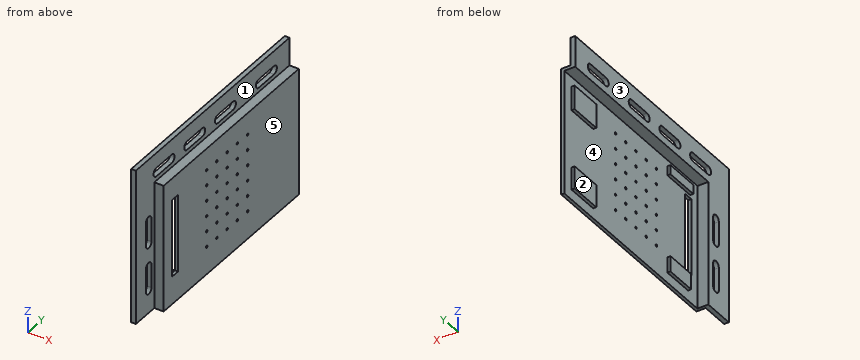
from build123d import *

# Parameters (mm, degrees)
EXTRUDE_1_DEPTH             = 3
EXTRUDE_2_DEPTH             = 6
EXTRUDE_3_DEPTH             = 3
SKETCH_5_W                  = 2
SKETCH_5_H                  = 80
EXTRUDE_4_DEPTH             = 130
SKETCH_6_W                  = 50
SKETCH_6_H                  = 6
CUT_EXTRUDE_1_DEPTH         = 130
SKETCH_7_W                  = 14.471008782
SKETCH_7_H                  = 21.149935912
SKETCH_7_W_2                = 15.39863755
SKETCH_7_W_3                = 10.018390695
SKETCH_7_H_2                = 20.222307144
SKETCH_7_W_4                = 5.936824115
SKETCH_7_H_3                = 22.263090434
EXTRUDE_5_DEPTH             = 2
SKETCH_8_R                  = 0.75
CUT_EXTRUDE_2_DEPTH         = 2
PATTERN_LINEAR_1_COUNT      = 5
PATTERN_LINEAR_1_PITCH      = 10
PATTERN_LINEAR_1_COUNT_DIR2 = 6
PATTERN_LINEAR_1_PITCH_DIR2 = 10


with BuildPart() as part:
    # Sketch 1 → Extrude 1 (new body)
    with BuildSketch(Plane(origin=(0, 0, 0), x_dir=(0, 0, -1), z_dir=(1, 0, 0))):
        Polygon((0, 0), (0, 150), (18, 150), (18, 18), (100, 18), (100, 0), align=None)
        with BuildLine():
            ThreePointArc((85, 9.75), (87.75, 12.5), (85, 15.25))
            Line((85, 15.25), (70, 15.25))
            ThreePointArc((70, 15.25), (67.25, 12.5), (70, 9.75))
            Line((70, 9.75), (85, 9.75))
        make_face(mode=Mode.SUBTRACT)
        with BuildLine():
            ThreePointArc((55, 9.75), (57.75, 12.5), (55, 15.25))
            Line((55, 15.25), (40, 15.25))
            ThreePointArc((40, 15.25), (37.25, 12.5), (40, 9.75))
            Line((40, 9.75), (55, 9.75))
        make_face(mode=Mode.SUBTRACT)
        with BuildLine():
            ThreePointArc((15.25, 135), (12.5, 137.75), (9.75, 135))
            Line((9.75, 135), (9.75, 120))
            ThreePointArc((9.75, 120), (12.5, 117.25), (15.25, 120))
            Line((15.25, 120), (15.25, 135))
        make_face(mode=Mode.SUBTRACT)
        with BuildLine():
            ThreePointArc((15.25, 95), (12.5, 97.75), (9.75, 95))
            Line((9.75, 95), (9.75, 80))
            ThreePointArc((9.75, 80), (12.5, 77.25), (15.25, 80))
            Line((15.25, 80), (15.25, 95))
        make_face(mode=Mode.SUBTRACT)
        with BuildLine():
            ThreePointArc((15.25, 65), (12.5, 67.75), (9.75, 65))
            Line((9.75, 65), (9.75, 50))
            ThreePointArc((9.75, 50), (12.5, 47.25), (15.25, 50))
            Line((15.25, 50), (15.25, 65))
        make_face(mode=Mode.SUBTRACT)
        with BuildLine():
            ThreePointArc((15.25, 35), (12.5, 37.75), (9.75, 35))
            Line((9.75, 35), (9.75, 20))
            ThreePointArc((9.75, 20), (12.5, 17.25), (15.25, 20))
            Line((15.25, 20), (15.25, 35))
        make_face(mode=Mode.SUBTRACT)
    extrude(amount=EXTRUDE_1_DEPTH)



with BuildPart() as body_2:
    # Sketch 2 → Extrude 2 (new body)
    with BuildSketch(Plane(origin=(3, 0, 0), x_dir=(0, 0, -1), z_dir=(1, 0, 0))):
        Polygon((18, 150), (20, 150), (20, 20), (100, 20), (100, 18), (20, 18), (18, 18), align=None)
    extrude(amount=EXTRUDE_2_DEPTH)


with BuildPart() as part_1:
    add(part.part)

    add(body_2.part)  # Extrude 3 merges body 2
    # Sketch 4 → Extrude 3 (add)
    with BuildSketch(Plane.ZY.offset(-3)):
        Polygon((-18, 18), (-18, 150), (-20, 150), (-20, 20), (-100, 20), (-100, 18), align=None)
    extrude(amount=EXTRUDE_3_DEPTH)

    # Sketch 5 → Extrude 4 (add)
    with BuildSketch(Plane(origin=(0, 20, 0), x_dir=(1, 0, 0), z_dir=(0, 1, 0))):
        with Locations((8, 60)):
            Rectangle(SKETCH_5_W, SKETCH_5_H)
    extrude(amount=EXTRUDE_4_DEPTH)

    # Sketch 6 → Cut-Extrude 1 (cut)
    with BuildSketch(Plane.ZY.offset(-7)):
        with Locations((-57, 29)):
            Rectangle(SKETCH_6_W, SKETCH_6_H)
    extrude(amount=-CUT_EXTRUDE_1_DEPTH, mode=Mode.SUBTRACT)

    # Sketch 7 → Extrude 5 (add)
    with BuildSketch(Plane.ZY.offset(-7)):
        with Locations((-86.256785513, 132.445159505)):
            Rectangle(SKETCH_7_W, SKETCH_7_H)
        with Locations((-34.031285871, 132.445159505)):
            Rectangle(SKETCH_7_W_2, SKETCH_7_H)
        with Locations((-88.483094557, 39.218468314)):
            Rectangle(SKETCH_7_W_3, SKETCH_7_H_2)
        with Locations((-27.074070111, 38.198076669)):
            Rectangle(SKETCH_7_W_4, SKETCH_7_H_3)
    extrude(amount=EXTRUDE_5_DEPTH)

    # Sketch 8 → Cut-Extrude 2 (cut)
    with BuildSketch(Plane.ZY.offset(-7)):
        with Locations((-82, 100)):
            Circle(SKETCH_8_R)
    cut_extrude_2 = extrude(amount=-CUT_EXTRUDE_2_DEPTH, mode=Mode.SUBTRACT)

    # Pattern Linear 1: Cut-Extrude 2 5 × 6
    with Locations(*[(0, -i * PATTERN_LINEAR_1_PITCH, j * PATTERN_LINEAR_1_PITCH_DIR2) for i in range(PATTERN_LINEAR_1_COUNT) for j in range(PATTERN_LINEAR_1_COUNT_DIR2) if (i, j) != (0, 0)]):
        add(cut_extrude_2, mode=Mode.SUBTRACT)


solid = part_1.part
Geometry: final body of the model. Coordinates: model frame, mm. Face numbers are marked on the shaded views. A direction names the side the tool comes from. Round coordinates to 2 decimals unless told otherwise and drop trailing zeros. Loops run counter-clockwise (first coordinate to the right, second up) from the corner with the lowest first, then second, coordinate; pieces in that order, holes last. Notation, with made-up numbers: M 52,-17.5 L 70,-17.5 A16 cw 70,-0.5 Z; hole C -5,-37 d11. An arc over 180 degrees is marked long. One line per question, with ' | ' between items.
(1) Cut plane B-B on y = 12.5. Return the cut outline in (x, z), plus the area to 3 significant figures.
Check result:
outline: M 0,-100 L 3,-100 L 3,-87.75 L 0,-87.75 Z; M 0,-67.25 L 3,-67.25 L 3,-57.75 L 0,-57.75 Z; M 0,-37.25 L 3,-37.25 L 3,0 L 0,0 Z | area: 177 mm2
(2) Cut plane D-D on y = 123.5. Return the cut outline in (x, z).
Check result:
outline: M 0,-20 L 7,-20 L 7,-26.33 L 5,-26.33 L 5,-41.73 L 7,-41.73 L 7,-79.02 L 5,-79.02 L 5,-93.49 L 7,-93.49 L 7,-100 L 9,-100 L 9,-18 L 3,-18 L 3,-15.25 L 0,-15.25 Z; M 0,-9.75 L 3,-9.75 L 3,0 L 0,0 Z
(3) Material intervals for line 1 along Z through (x, y) = (6, 129); line 2 along Y through (x, z) = (5.25, -84); line 3 along Y through (x, z) = (5.75, -35.5), sorted ascending. Write a range as from..to.
Check result:
line 1: z = -93.49..-79.02, -41.73..-26.33, -20..-18 | line 2: y = 18..20, 29.11..49.33, 121.87..143.02 | line 3: y = 18..20, 121.87..143.02
(4) Access query for the marked faces 1, 2 and 3. Directions: +Z, -Z, +X, -X, +Y, -Y. A direction counts if a zero-diameter tool reaches every point of the face in a straight line with its end or side. Return the directions, or none.
Check result:
face 1: +Z, +X, -Y | face 2: -Z, -X, +Y | face 3: +Z, -Z, -X, +Y, -Y
(5) Cut plane C-C on y = 72.5. Return the cut outline in (x, z), plus the area to 3 significant figures.
Check result:
outline: M 0,-20 L 7,-20 L 7,-100 L 9,-100 L 9,-18 L 3,-18 L 3,0 L 0,0 Z | area: 232 mm2
(6) Cut plane A-A on z = -75. Return the cut outline in (x, y).
Check result:
outline: M 0,0 L 3,0 L 3,9.75 L 0,9.75 Z; M 0,15.25 L 3,15.25 L 3,18 L 9,18 L 9,26 L 7,26 L 7,20 L 0,20 Z; M 7,32 L 9,32 L 9,150 L 7,150 Z
(7) Pull-direction query (Z, two-part tool) for the marked faces 4 and 5; classes: +Z half, -Z half, draft (parallel to the pull), parting line (faces both ways), or undercut.
Check result:
face 4: undercut | face 5: draft
(8) Contact query for flat-ended pins moving along their axis: P1, Ø2, axis at x = 6.5, y = 129.5, coming from the +Z side; P2, Ø2, axis at y = 92, z = -52.5, coming from the -X side; P3, Ø4.5, axis at y = 133.5, z = -36, coming from the -X side. Output: stop coordinate, or through.
Check result:
P1: stops at z = -18 | P2: stops at x = 7 | P3: stops at x = 5
